Source: CAD feature listing. Evaluate the final solid. Frame: model axes, mm. Coordinates: 2 decimals unless noted, no trailing zeros. One line per question, with ' | ' between items.
from build123d import *

# Parameters (mm, degrees)
SKETCH1_W           = 3
SKETCH1_H           = 30
BOSS_EXTRUDE1_DEPTH = 3


with BuildPart() as part:
    # Sketch1 → Boss-Extrude1 (new body)
    with BuildSketch(Plane(origin=(0, 0, 0), x_dir=(1, 0, 0), z_dir=(0, 1, 0))):
        Polygon((31, 0), (42, 0), (42, 404), (31, 404), (31, 407), (11, 407), (11, 404), (0, 404), (0, 0), (11, 0), (11, -3), (31, -3), align=None)
        with Locations((37.5, 344)):
            Rectangle(SKETCH1_W, SKETCH1_H, mode=Mode.SUBTRACT)
        with Locations((37.5, 197)):
            Rectangle(SKETCH1_W, SKETCH1_H, mode=Mode.SUBTRACT)
        with Locations((37.5, 55)):
            Rectangle(SKETCH1_W, SKETCH1_H, mode=Mode.SUBTRACT)
        with Locations((4.5, 55)):
            Rectangle(SKETCH1_W, SKETCH1_H, mode=Mode.SUBTRACT)
        with Locations((4.5, 197)):
            Rectangle(SKETCH1_W, SKETCH1_H, mode=Mode.SUBTRACT)
        with Locations((4.5, 344)):
            Rectangle(SKETCH1_W, SKETCH1_H, mode=Mode.SUBTRACT)
    extrude(amount=BOSS_EXTRUDE1_DEPTH)


solid = part.part
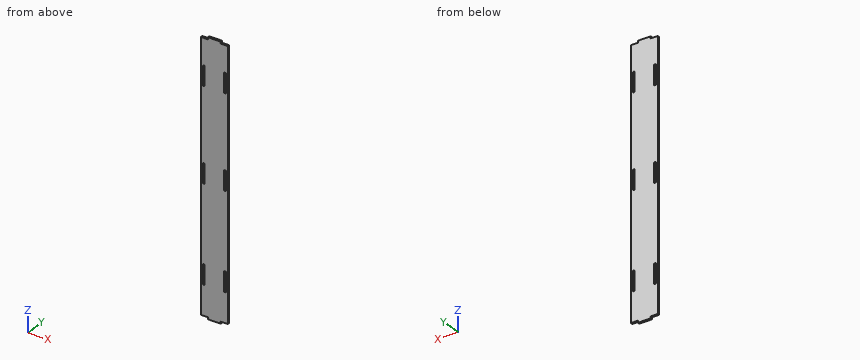
(1) Cut plane A-A (y = 2). State how many separate pieces and enclosed holes the cut face has, and give its area (3 significant figures).
Taken from the geometry:
separate pieces: 1 | enclosed holes: 6 | area: 16,500 mm²
(2) Material intervals for L1, parallel to X at y = 2.1, z = -334; L2, parallel to Z at x = 9, y = 0.2, sorted ascending. Write a range as from..to.
Taken from the geometry:
L1: x = 0..3, 6..36, 39..42 | L2: z = -404..0
(3) Pin query (flat end, axial travel): P1, Ø1.5, axis at x = 4.5, y = 1, coming from the -Z side. Return the tip coordinate at first contact, or that it passes through.
Taken from the geometry:
P1: stops at z = -404
